Input: part model. Units: mm. Frame: model coordinates. Coordinates: 2 decimals unless noted, no trailing zeros. Loops run counter-clockwise (first coordinate to the right, second up) from the corner with the lowest first, then second, coordinate; pieces in that order, holes last.
Item 1: Section B-B on x = 32.5. Return loops of the section in (y, z), and give its area (3 significant figures).
Item 2: Section A-A on z = 1.75. Return loops of the section in (x, y), and give its area (3 significant figures).
Item 3: Ray query, line 1 along Y through (x, z) = (-7, 1); line 2 along Y through (x, z) = (1.5, 0.9); line 3 along X through (y, z) = (2.75, 3.05). Return the intervals inside material, ascending.
Item 4: Section C-C on y = -3. Return loops of the section in (x, z).
Item 5: Contact query for a flat-ended pin moving along its axis: P1, Ø2, axis at x = -6.5, y = 1, coming from the -Z side. Output: stop coordinate, or through.
Item 6: Section D-D on x = -9. Return loops of the section in (y, z).
```python
from build123d import *

# Parameters (mm, degrees)
SKETCH1_W           = 52
SKETCH1_H           = 16
SKETCH1_R           = 2
BOSS_EXTRUDE1_DEPTH = 4
FILLET1_R           = 1
CUT_EXTRUDE1_DEPTH  = 3


with BuildPart() as part:
    # Sketch1 → Boss-Extrude1 (new body)
    with BuildSketch(Plane.XY):
        with Locations((13.855253101, 1.7017189)):
            Rectangle(SKETCH1_W, SKETCH1_H)
        with Locations((-5.644746899, -0.2982811)):
            Circle(SKETCH1_R, mode=Mode.SUBTRACT)
        with Locations((33.355253101, -0.2982811)):
            Circle(SKETCH1_R, mode=Mode.SUBTRACT)
    extrude(amount=BOSS_EXTRUDE1_DEPTH)

    # Fillet1
    fillet1_edges = [part.edges().sort_by_distance(p)[0] for p in [
        (39.855253101, 1.7017189, 4),
        (13.855253101, 9.7017189, 4),
        (-12.144746899, 1.7017189, 4),
        (13.855253101, 9.7017189, 0),
        (39.855253101, 1.7017189, 0),
        (13.855253101, -6.2982811, 0),
        (-12.144746899, 1.7017189, 0),
        (13.855253101, -6.2982811, 4),
        (-12.144746899, 9.7017189, 2),
        (39.855253101, 9.7017189, 2),
        (39.855253101, -6.2982811, 2),
        (-12.144746899, -6.2982811, 2),
    ]]
    fillet(fillet1_edges, radius=FILLET1_R)

    # Sketch5 → Cut-Extrude1 (cut)
    with BuildSketch(Plane(origin=(0, 0, 0), x_dir=(-1, 0, 0), z_dir=(0, 0, -1))):
        Polygon((-29.025126082, -0.2982811), (-31.190189592, 3.4517189), (-35.520316611, 3.4517189), (-37.68538012, -0.2982811), (-35.520316611, -4.0482811), (-31.190189592, -4.0482811), align=None)
        Polygon((1.31461988, -0.2982811), (3.479683389, -4.0482811), (7.809810408, -4.0482811), (9.974873918, -0.2982811), (7.809810408, 3.4517189), (3.479683389, 3.4517189), align=None)
    extrude(amount=-CUT_EXTRUDE1_DEPTH, mode=Mode.SUBTRACT)


solid = part.part
```
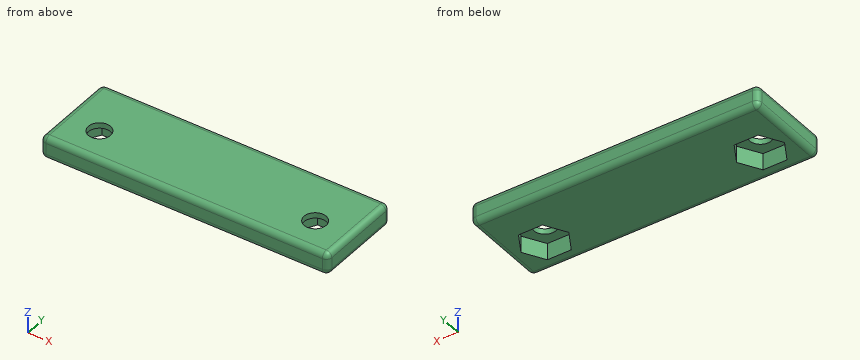
Results found:
1. outline: (-6.3, 1) arc R1 ccw to (-5.3, 0) - (-4.05, 0) - (-4.05, 3) - (-2.11, 3) - (-2.11, 4) - (-5.3, 4) arc R1 ccw to (-6.3, 3) - close; (1.51, 3) - (3.45, 3) - (3.45, 0) - (8.7, 0) arc R1 ccw to (9.7, 1) - (9.7, 3) arc R1 ccw to (8.7, 4) - (1.51, 4) - close
1. area: 37.0 mm2
2. outline: (-12.14, -5.3) arc R1 ccw to (-11.14, -6.3) - (38.86, -6.3) arc R1 ccw to (39.86, -5.3) - (39.86, 8.7) arc R1 ccw to (38.86, 9.7) - (-11.14, 9.7) arc R1 ccw to (-12.14, 8.7) - close; hole (-9.97, -0.3) - (-7.81, -4.05) - (-3.48, -4.05) - (-1.31, -0.3) - (-3.48, 3.45) - (-7.81, 3.45) - close; hole (29.03, -0.3) - (31.19, -4.05) - (35.52, -4.05) - (37.69, -0.3) - (35.52, 3.45) - (31.19, 3.45) - close
2. area: 734 mm2
3. line 1: y = -6.3 to -4.05, 3.45 to 9.7
3. line 2: y = -6.29 to 9.7
3. line 3: x = -12.14 to 39.85
4. outline: (-12.14, 1) arc R1 ccw to (-11.14, 0) - (-8.42, 0) - (-8.42, 3) - (-2.87, 3) - (-2.87, 0) - (30.58, 0) - (30.58, 3) - (36.13, 3) - (36.13, 0) - (38.86, 0) arc R1 ccw to (39.86, 1) - (39.86, 3) arc R1 ccw to (38.86, 4) - (-11.14, 4) arc R1 ccw to (-12.14, 3) - close
5. P1: stops at z = 3
6. outline: (-6.3, 1) arc R1 ccw to (-5.3, 0) - (-1.99, 0) - (-1.99, 3) - (1.39, 3) - (1.39, 0) - (8.7, 0) arc R1 ccw to (9.7, 1) - (9.7, 3) arc R1 ccw to (8.7, 4) - (-5.3, 4) arc R1 ccw to (-6.3, 3) - close
